Autodesk Inventor part; units mm, degrees
ref_plane "YZ Plane" through (0, 0, 0) normal (1, 0, 0) x (0, 1, 0)
ref_plane "XZ Plane" through (0, 0, 0) normal (0, 1, 0) x (-1, 0, 0)
ref_plane "XY Plane" through (0, 0, 0) normal (0, 0, 1) x (1, 0, 0)
sketch "Sketch1" plane through (0, 0, 0) normal (0, 0, 1) x (1, 0, 0)
  circle A0 centre (0, 0) radius 7.3025
  dimension "d0" = 14.605
extrude "Extrusion1" add sketch "Sketch1" along normal blind 421.005
sketch "Sketch2" plane through (0, 0, 421.005) normal (0, 0, 1) x (1, 0, 0)
  circle A0 centre (0, 0) radius 9.017
  circle A1 centre (0, 0) radius 12.7
  dimension "d3" = 18.034
  dimension "d4" = 25.4
extrude "Extrusion2" add sketch "Sketch2" against normal blind 457.2
sketch "Sketch3" plane through (0, 0, 421.005) normal (0, 0, 1) x (1, 0, 0)
  circle A0 centre (0, 0) radius 7.3025
  circle A1 centre (0, 0) radius 12.7
  circle A2 centre (0, 0) radius 8.9258
extrude "Extrusion3" cut sketch "Sketch3" against normal blind 508 contours A1
sketch "Sketch5" plane through (0, 0, 421.005) normal (0, 0, 1) x (1, 0, 0)
  circle A0 centre (0, 0) radius 38.1
  dimension "d12" = 76.2
extrude "Extrusion5" add sketch "Sketch5" against normal blind 337.5025
sketch "Sketch7" plane through (0, 0, 421.005) normal (0, 0, 1) x (1, 0, 0)
  circle A0 centre (0, 0) radius 7.3768
  circle A1 centre (0, 0) radius 38.1
extrude "Extrusion6" cut sketch "Sketch7" against normal blind 83.5025
sketch "Sketch9" plane through (0, 0, 421.005) normal (0, 0, 1) x (1, 0, 0)
  circle A0 centre (0, 0) radius 7.3025
  circle A1 centre (0, 0) radius 10.3013
extrude "Extrusion7" cut sketch "Sketch9" against normal blind 58.1025 contours A0 | A1
properties part number "Conveyor Axle"
Geometry check sheet. Reference: the model listing, model coordinates, mm. A direction names the side the tool comes from. Give positions to 0.01 mm unless a question says otherwise; leave off trailing zeros. Order: outer loops, then holes, each group sorted by start corner. A loop starts at its lowest first (then second) coordinate and runs counter-clockwise, first axis right, second up. Notation, with made-up numbers: (18.25, 17) - (48.25, 17) arc R21 ccw to (48.25, 50) - close; hole circle Ø1 at (45.5, -40). An arc over 180 degrees is marked (long way). Use one line per item in the form item = value.
1) Access from +Z, -Z, +X, -X, +Y, -Y to the whole of each face (thin tool, end or side, straight path). Record for faces 1 (the face through (0, 0, 362.902)), 2 (the face through (-5.854, -4.489, 350.38)), 3 (the face through (-5.38, -4.94, 41.17)).
Working result:
face_1 = +Z, +X, -X, +Y, -Y
face_2 = +Z
face_3 = -Z
2) Sectioned sample at A-A (x = 0). Record the boundary of the cut face in (y, z).
Working result:
outline = (-38.1, 83.5) - (-7.3, 83.5) - (-7.3, 0) - (7.3, 0) - (7.3, 83.5) - (38.1, 83.5) - (38.1, 337.5) - (7.38, 337.5) - (7.38, 362.9) - (-7.38, 362.9) - (-7.38, 337.5) - (-38.1, 337.5) - close
3) Sectioned sample at D-D (z = 55). Record the boundary of the cut face in (x, y) (1 decimal), and give its area (3 significant figures).
Working result:
outline = circle Ø14.6 at (0, 0)
area = 168 mm^2
4) Depth check by flat-ended pin: pin 1 Ø10 at (y, z) = (14, 99) entering from +X; pin 2 Ø2 at (x, z) = (24.5, 238.5) entering from -Y; pin 3 Ø2 at (x, y) = (23, -1.5) entering from -Z. Enter the tip coordinate at first touch or a pass-through.
Working result:
pin_1 = 37.02
pin_2 = -29.99
pin_3 = 83.5
5) Sectioned sample at C-C (z = 128). Record the boundary of the cut face in (x, y), and give its area (3 significant figures).
Working result:
outline = circle Ø76.2 at (0, 0)
area = 4,560 mm^2
6) Material ranges on probe 1 along Z at (x, y) = (-7, 15); probe 2 along Y at (x, z) = (0, 156); probe 3 along X at (y, z) = (-3, 181), recorded low to high. Write a range as from..to.
Working result:
probe_1 = 83.5..337.5
probe_2 = -38.1..38.1
probe_3 = -37.98..37.98
